Verification items for the finished model (mm, model axes). A direction names the side the tool comes from. Round coordinates to 2 decimals unless told otherwise and drop trailing zeros. Write each loop counter-clockwise with the first axis right and the second up, starting at its lowest first coordinate (ties: lowest second). Pieces come first, ordered by that corner, then holes. Notation, with made-up numbers: M 14.5,-38.5 L 42.5,-38.5 A26 ccw 42.5,-5.5 Z; hole C 27,-12.75 d6. An arc over 180 degrees is marked long. Answer in a Markdown table with one row per item. Add a question column.
1. Sectioned sample at C-C on y = 13.5. Record the cut outline in (x, z), plus the area to 3 significant figures.
2. Sectioned sample at B-B on z = -15. Record the cut outline in (x, y).
3. Set-up check for faces 4 (the flat face through (6, 1, -18)), 5 (the flat face through (64, 1, -12)), 6 (the flat face through (0, 1, -6)), 7 (the cylindrical face through (48.788, 69.234, -16.847)): record each of +Z, -Z, +X, -X, +Y, -Y from which the full face is reachable in a straight line by a thin tool's end or side.
4. Material ranges on probe 1 along X at (y, z) = (64.5, -15); probe 2 along Y at (x, z) = (49.4, -15); probe 3 along Y at (x, z) = (11, -18.5), recorded low to high.
5. Go/stop test with flat-tipped pins: pin 1 Ø3 at (x, z) = (16.5, -4) entering from +Y; pin 2 Ø3 at (x, y) = (40.5, 25.5) entering from -Z; pin 3 Ø4 at (x, y) = (23, 9) entering from -Z; pin 4 Ø0.9 at (x, y) = (6, 1.5) entering from +Z. Record where each tip stops, or that it passes through.
6. Sectioned sample at A-A on x = 65. Record the cut outline in (y, z), plus the area to 3 significant figures.
7. Draft check along Z on faces 1 (the cylindrical face through (57, 1, -15)), 2 (the cylindrical face through (69.4, 1.48, -0.57)), 3 (the flat face through (35, 0, -15)). Enter one of: pulls with the +Z half, pulls with the -Z half, needs draft (parallel to the pull), parting line crosses it, or undercut.
8. Sectioned sample at D-D on x = 54. Record the cut outline in (y, z).
```python
from build123d import *

# Parameters (mm, degrees)
BOSS_EXTRUDE2_DEPTH = 3
SKETCH3_R           = 15
BOSS_EXTRUDE3_DEPTH = 5
SKETCH4_R           = 15
SKETCH4_R_2         = 12.7
BOSS_EXTRUDE5_DEPTH = 75
SKETCH5_R           = 2
CUT_EXTRUDE1_DEPTH  = 40


with BuildPart() as part:
    # Sketch1 → Boss-Extrude2 (new body)
    with BuildSketch(Plane(origin=(0, 0, 0), x_dir=(1, 0, 0), z_dir=(0, 1, 0))):
        with BuildLine():
            Line((2, 0), (68, 0))
            ThreePointArc((68, 0), (69.414213562, 0.585786438), (70, 2))
            Line((70, 2), (70, 10))
            ThreePointArc((70, 10), (69.414213562, 11.414213562), (68, 12))
            Line((68, 12), (60, 12))
            ThreePointArc((60, 12), (57, 15), (60, 18))
            Line((60, 18), (68, 18))
            ThreePointArc((68, 18), (69.414213562, 18.585786438), (70, 20))
            Line((70, 20), (70, 28))
            ThreePointArc((70, 28), (69.414213562, 29.414213562), (68, 30))
            Line((68, 30), (2, 30))
            ThreePointArc((2, 30), (0.585786438, 29.414213562), (0, 28))
            Line((0, 28), (0, 20))
            ThreePointArc((0, 20), (0.585786438, 18.585786438), (2, 18))
            Line((2, 18), (10, 18))
            ThreePointArc((10, 18), (13, 15), (10, 12))
            Line((10, 12), (2, 12))
            ThreePointArc((2, 12), (0.585786438, 11.414213562), (0, 10))
            Line((0, 10), (0, 2))
            ThreePointArc((0, 2), (0.585786438, 0.585786438), (2, 0))
        make_face()
    extrude(amount=BOSS_EXTRUDE2_DEPTH)

    # Sketch3 → Boss-Extrude3 (add)
    with BuildSketch(Plane(origin=(0, 3, 0), x_dir=(1, 0, 0), z_dir=(0, 1, 0))):
        with Locations(Location((35, 15, 0), (0, 0, 270))):
            Circle(SKETCH3_R)
    extrude(amount=BOSS_EXTRUDE3_DEPTH)

    # Sketch4 → Boss-Extrude5 (add)
    with BuildSketch(Plane(origin=(0, 8, 0), x_dir=(1, 0, 0), z_dir=(0, 1, 0))):
        with Locations(Location((35, 15, 0), (0, 0, 270))):
            Circle(SKETCH4_R)
        with Locations(Location((35, 15, 0), (0, 0, 270))):
            Circle(SKETCH4_R_2, mode=Mode.SUBTRACT)
    extrude(amount=BOSS_EXTRUDE5_DEPTH)

    # Sketch5 → Cut-Extrude1 (cut)
    with BuildSketch(Plane(origin=(70, 0, 0), x_dir=(0, 0, -1), z_dir=(1, 0, 0))):
        with Locations((15, 70)):
            Circle(SKETCH5_R)
    extrude(amount=-CUT_EXTRUDE1_DEPTH, mode=Mode.SUBTRACT)


solid = part.part
```
Geometry check:
| question | item | result |
|---|---|---|
| 1 | outline | C 35,-15 d30; hole C 35,-15 d25.4 |
| 1 | area | 200 mm2 |
| 2 | outline | M 13,0 L 57,0 L 57,3 L 50,3 L 50,68 L 47.7,68 L 47.7,8 L 22.3,8 L 22.3,83 L 20,83 L 20,3 L 13,3 Z; M 47.7,72 L 50,72 L 50,83 L 47.7,83 Z |
| 3 | face 4 | -X, +Y, -Y |
| 3 | face 5 | +X, +Y, -Y |
| 3 | face 6 | +Z, -Z, -X, +Y, -Y |
| 3 | face 7 | +X |
| 4 | probe 1 | x = 20 to 22.3, 47.7 to 50 |
| 4 | probe 2 | y = 0 to 68, 72 to 83 |
| 4 | probe 3 | y = 0 to 3 |
| 5 | pin 1 | stops at y = 3 |
| 5 | pin 2 | stops at z = -29.46 |
| 5 | pin 3 | stops at z = -26.18 |
| 5 | pin 4 | stops at z = 0 |
| 6 | outline | M 0,-30 L 3,-30 L 3,-18 L 0,-18 Z; M 0,-12 L 3,-12 L 3,0 L 0,0 Z |
| 6 | area | 72.0 mm2 |
| 7 | face 1 | undercut |
| 7 | face 2 | pulls with the +Z half |
| 7 | face 3 | needs draft |
| 8 | outline | M 0,-30 L 3,-30 L 3,0 L 0,0 Z |
